The model under review builds one solid part; all positions refer to its coordinate system, in mm. A direction names the side the tool comes from. Round coordinates to 2 decimals unless told otherwise and drop trailing zeros. Order: outer loops, then holes, each group sorted by start corner. A loop starts at its lowest first (then second) coordinate and runs counter-clockwise, first axis right, second up. Notation, with made-up numbers: (53, 64.5) -> (92, 64.5) arc R21 ccw to (92, 76.5) -> close; hole circle Ø6 at (-23.75, 6.5). An arc over 180 degrees is marked (long way). Use a Markdown table: item, result. Add a question column.
```python
from build123d import *

# Parameters (mm, degrees)
F1_DEPTH = 63.5
F2_DEPTH = 25.4
F3_DEPTH = 7.9375
F5_R     = 6.35


with BuildPart() as f1:
    # F0 (on Front) → F1 (new body, symmetric)
    with BuildSketch(Plane.XZ):
        Polygon((22.225, 9.525), (-41.275, 9.525), (-41.275, -9.525), (41.275, -9.525), (41.275, 9.525), align=None)
    extrude(amount=F1_DEPTH, both=True)

    # F0 (on Front) → F2 (join, symmetric)
    with BuildSketch(Plane.XZ):
        with BuildLine():
            Line((22.225, 27.0002), (22.225, 9.525))
            Line((22.225, 9.525), (41.275, 9.525))
            Line((41.275, 9.525), (41.275, 27.0002))
            ThreePointArc((41.275, 27.0002), (45.9246798487, 38.2255201513), (57.15, 42.8752))
            Line((57.15, 42.8752), (60.325, 42.8752))
            Line((60.325, 42.8752), (60.325, 61.9252))
            Line((60.325, 61.9252), (57.15, 61.9252))
            add(Edge.make_bspline(
                [(56.2807505005, 61.9143809342), (56.5712025295, 61.918597831), (56.8609603005, 61.9222027986), (57.15, 61.9252)],
                knots=[110.7360058155, 110.7360058155, 110.7360058155, 110.7360058155, 111.5045361635, 111.5045361635, 111.5045361635, 111.5045361635], degree=3))
            ThreePointArc((56.2807505005, 61.9143809342), (32.1488583884, 51.3866417887), (22.225, 27.0002))
        make_face()
        Polygon((85.8728378947, 61.9252), (60.325, 61.9252), (60.325, 42.8752), (85.7546306228, 42.8752), align=None)
    extrude(amount=F2_DEPTH, both=True)

    # F0 (on Front) → F3 (join, symmetric)
    with BuildSketch(Plane.XZ):
        with BuildLine():
            add(Edge.make_bspline(
                [(-41.275, 9.525), (-41.8342912286, 47.9946959392), (14.430096654, 61.3067766904), (56.2807505005, 61.9143809342)],
                knots=[0, 0, 0, 0, 110.7360058155, 110.7360058155, 110.7360058155, 110.7360058155], degree=3))
            Line((-41.275, 9.525), (22.225, 9.525))
            Line((22.225, 9.525), (22.225, 27.0002))
            ThreePointArc((22.225, 27.0002), (32.1488583884, 51.3866417887), (56.2807505005, 61.9143809342))
        make_face()
    extrude(amount=F3_DEPTH, both=True)

    # F0 (on Front) → F4 (revolve)
    with BuildSketch(Plane.XZ):
        Polygon((85.9023109078, 66.675), (85.8728378947, 61.9252), (85.7546306228, 42.8752), (85.725, 38.1), (111.125, 38.1), (111.125, 66.675), align=None)
    revolve(axis=Axis((85.8136554539, 0, 52.3875), (0.0062049867, 0, 0.9999807489)))

    # F5
    f5_edges = [f1.edges().sort_by_distance(p)[0] for p in [
        (41.275, -63.5, 0),
        (41.275, 63.5, 0),
        (-41.275, 63.5, 0),
        (-41.275, -63.5, 0),
    ]]
    fillet(f5_edges, radius=F5_R)


solid = f1.part
```
Q1. Add section B-B, the plane y = -40. Give the boundary of the cut face in (x, z) (3 decimals).
Q2. Draft analysis for pull direction X (two halves, no side actions). For faces 4 (the face through (60, 0, 42.875)), 5 (the face through (32.414, 16.547, 51.656)), 6 (the face through (47, -25.4, 42)), state which applies: released by +X, released by -X, zero draft, split by the parting line, or undercut.
Q3. For faces 1 (the face through (45.8, -0.4, 38.1)), 2 (the face through (60, -2, 61.925)), 3 (the face through (22.225, 17, 18)), list the 3-axis set-ups (+Z, -Z, +X, -X, +Y, -Y) from which the entire face can be reached by the end or side of a thin tool; tool diameter is ignored.
Q4. To check wall thickness, follow line 1 along Z through (x, y) = (15, -13) (3 decimals); line 2 along Y through (x, z) = (21, 49.5); line 3 along Z through (x, y) = (87.5, -3.5). State the ranges of each line that lie inside material, in increasing order.
Q5. For pin 1 (10 mm diameter, centred on y = -1, z = 45.5, fed in from -X); pin 2 (14.5 mm diameter, centred on x = 73.5, y = 2.5, fed in from -Z); pin 3 (4 mm diameter, centred on x = 32, y = -39.5, fed in from +Z) (3 decimals), all flat-tipped, find the tip position at first contact; note any pin that passes through.
Q6. Add section A-A, the plane z = 0. Give the boundary of the cut face in (x, y) (3 decimals).
Return value:
| question | item | result |
|---|---|---|
| 1 | outline | (-41.275, -9.525) -> (41.275, -9.525) -> (41.275, 9.525) -> (-41.275, 9.525) -> close |
| 2 | face 4 | undercut |
| 2 | face 5 | released by -X |
| 2 | face 6 | zero draft |
| 3 | face 1 | -Z, +Y, -Y |
| 3 | face 2 | +Z, -X |
| 3 | face 3 | +Z, -X, +Y |
| 4 | line 1 | -9.525 to 9.525 |
| 4 | line 2 | -7.94 to 7.94 |
| 4 | line 3 | 38.11 to 66.69 |
| 5 | pin 1 | x = -24.98 |
| 5 | pin 2 | z = 38.16 |
| 5 | pin 3 | z = 9.525 |
| 6 | outline | (-41.275, -57.15) arc R6.35 ccw to (-34.925, -63.5) -> (34.925, -63.5) arc R6.35 ccw to (41.275, -57.15) -> (41.275, 57.15) arc R6.35 ccw to (34.925, 63.5) -> (-34.925, 63.5) arc R6.35 ccw to (-41.275, 57.15) -> close |
